```python
from build123d import *

# Parameters (mm, degrees)
EXTRUDE_1_DEPTH       = 177.5
EXTRUDE_2_DEPTH       = 109
EXTRUDE_3_DEPTH       = 2
SKETCH_5_W            = 355
SKETCH_5_H            = 250
SKETCH_5_W_2          = 353
SKETCH_5_H_2          = 248
CUT_EXTRUDE_1_DEPTH   = 2
SKETCH_6_W            = 343
SKETCH_6_H            = 207
CUT_EXTRUDE_1_2_DEPTH = 2
CHAMFER_1_SIZE        = 1.154
CHAMFER_1_SIZE2       = 1.998786632
SKETCH_7_R            = 3.5
CUT_EXTRUDE_2_DEPTH   = 0.5
FILLET_1_R            = 0.5
SKETCH_8_R            = 4
EXTRUDE_4_DEPTH       = 140.5


with BuildPart() as part:
    # 草图1 → 凸台-拉伸1 (new, symmetric)
    with BuildSketch(Plane(origin=(0, 0, 0), x_dir=(0, 0, -1), z_dir=(1, 0, 0))):
        Polygon((0, 0), (0, 255), (-5, 255), (-5, 5), align=None)
    extrude(amount=EXTRUDE_1_DEPTH, both=True)

    # 草图3 → 凸台-拉伸2 (add, symmetric)
    with BuildSketch(Plane(origin=(0, 0, 0), x_dir=(0, 0, -1), z_dir=(1, 0, 0))):
        Polygon((0, 0), (-6.583760775, -7.526891394), (-18.557046178, -8.32716426), (-18.557046178, -2.82716426), (-5, 5), align=None)
    extrude(amount=EXTRUDE_2_DEPTH, both=True)

    # 草图4 → 凸台-拉伸3 (add)
    with BuildSketch(Plane.XY.offset(5)):
        Polygon((-177.5, 255), (-177.5, 5), (-109, 5), (109, 5), (177.5, 5), (177.5, 255), align=None)
    extrude(amount=EXTRUDE_3_DEPTH)

    # 草图5 → Cut-Extrude 1 (cut)
    with BuildSketch(Plane.XY.offset(7)):
        with Locations((0, 130)):
            Rectangle(SKETCH_5_W, SKETCH_5_H)
        with Locations((0, 130)):
            Rectangle(SKETCH_5_W_2, SKETCH_5_H_2, mode=Mode.SUBTRACT)
    extrude(amount=-CUT_EXTRUDE_1_DEPTH, mode=Mode.SUBTRACT)

    # 草图6 → Cut-Extrude 1 2 (cut)
    with BuildSketch(Plane.XY.offset(7)):
        with Locations((0, 139.5)):
            Rectangle(SKETCH_6_W, SKETCH_6_H)
    extrude(amount=-CUT_EXTRUDE_1_2_DEPTH, mode=Mode.SUBTRACT)

    # 倒角1
    chamfer_1_edges = [part.edges().sort_by_distance(p)[0] for p in [
        (-171.5, 139.5, 7),
        (0, 36, 7),
        (171.5, 139.5, 7),
        (0, 243, 7),
    ]]
    chamfer_1_side = [part.faces().sort_by_distance(p)[0] for p in [
        (0, 10.314081594, 7),
    ]]
    chamfer(chamfer_1_edges, length=CHAMFER_1_SIZE, length2=CHAMFER_1_SIZE2, reference=chamfer_1_side[0])

    # 草图7 → 切除-拉伸2 (cut)
    with BuildSketch(Plane.XY.offset(7)):
        with Locations((0, 249)):
            Circle(SKETCH_7_R)
    extrude(amount=-CUT_EXTRUDE_2_DEPTH, mode=Mode.SUBTRACT)

    # 圆角1
    fillet_1_edges = [part.edges().sort_by_distance(p)[0] for p in [
        (-3.5, 249, 7),
    ]]
    fillet(fillet_1_edges, radius=FILLET_1_R - 0.0001)  # a hair under: the kernel refuses the full size

    # 草图8 → 凸台-拉伸4 (add, symmetric)
    with BuildSketch(Plane(origin=(0, 0, 0), x_dir=(0, 0, -1), z_dir=(1, 0, 0))):
        with Locations(Location((-10.557046178, -3.382641438, 0), (0, 0, 180))):
            Circle(SKETCH_8_R)
    extrude(amount=EXTRUDE_4_DEPTH, both=True)


solid = part.part
```
Source: CAD feature listing. Evaluate the final solid. Frame: model axes, mm. A direction names the side the tool comes from. Coordinates: 2 decimals unless noted, no trailing zeros. Loops run counter-clockwise (first coordinate to the right, second up) from the corner with the lowest first, then second, coordinate; pieces in that order, holes last. Notation, with made-up numbers: M 81,10 L 115,10 A13 cw 115,28 Z; hole C 25,-27.5 d2. An arc over 180 degrees is marked long. Use a Markdown table: item, result. Add a question column.
Q1. Section query C-C, the plane z = 10.25. Return loops of the section in (x, y).
Q2. Draft query along X for faces 1 (the flat face through (1.53, -7.92, 12.49)), 2 (the flat face through (0, 249, 6.5)), 3 (the flat face through (-109, 0, 7)). Return one class per face: pulls with the +X half, pulls with the -X half, needs draft (parallel to the pull), parting line crosses it, or undercut.
Q3. Access query for faces 4 (the flat face through (109, 0, 7)), 5 (the flat face through (-2, 141, 5)), 6 (the flat face through (-1, 30, 7)). Directions: +Z, -Z, +X, -X, +Y, -Y. A direction counts if a zero-diameter tool reaches every point of the face in a straight line with its end or side. Return the directions, or none.
Q4. First-contact query: pin 1 (4 mm diameter, centred on y = -1.5, z = 9, fed in from -X); pin 2 (1.6 mm diameter, centred on x = 5.5, z = 6, fed in from +Y); pin 3 (4 mm diameter, centred on y = -3, z = 13, fed in from +X); pin 4 (12 mm diameter, centred on x = -5, y = 93, fed in from -Z). Flat tips, straight axial feed; report the tip coordinate or a pass-through.
Q5. Material intervals for L1, parallel to X at y = 249, z = 6.55; L2, parallel to Z at x = -18, y = 32; L3, parallel to Z at x = -98.5, y = 76.5, sorted ascending.
Result:
| question | item | result |
|---|---|---|
| 1 | outline | M -140.5,-7.37 L -109,-7.37 L -109,-7.77 L 109,-7.77 L 109,-7.37 L 140.5,-7.37 L 140.5,0.61 L 109,0.61 L 109,1.97 L -109,1.97 L -109,0.61 L -140.5,0.61 Z |
| 2 | face 1 | needs draft |
| 2 | face 2 | undercut |
| 2 | face 3 | pulls with the -X half |
| 3 | face 4 | +X |
| 3 | face 5 | +Z |
| 3 | face 6 | +Z, +X, -X, +Y |
| 4 | pin 1 | stops at x = -140.5 |
| 4 | pin 2 | stops at y = 254 |
| 4 | pin 3 | stops at x = 140.5 |
| 4 | pin 4 | stops at z = 0 |
| 5 | L1 | x = -176.5 to -3.5, 3.5 to 176.5 |
| 5 | L2 | z = 0 to 7 |
| 5 | L3 | z = 0 to 5 |
